For this review, use the dimensioned drawing (mm, ordinates from the lowest corner) and the shaded views. A direction names the side the tool comes from. Coordinates: 2 decimals unless noted, no trailing zeros. Loops run counter-clockwise (first coordinate to the right, second up) from the corner with the lowest first, then second, coordinate; pieces in that order, holes last. Notation, with made-up numbers: (63, 47.5) - (111, 47.5) arc R28 cw to (111, 82.5) - close; hole circle Ø1 at (88.25, -8.75). An arc over 180 degrees is marked (long way). Use a Markdown table: item, result. Add a question column.
1) The part is to be moulded in two halves that separate along X. For the marked faces 1, 2 and 3, say which applies: pulls with the +X half, pulls with the -X half, needs draft (parallel to the pull), parting line crosses it, or undercut.
2) Add section C-C, the plane z = 8. Give the boundary of the cut face in (x, y), and give its area (3 significant figures).
3) Add section B-B, the plane y = 30. Give the boundary of the cut face in (x, z).
4) Add section D-D, the plane z = 21. Give the boundary of the cut face in (x, y).
5) Clearance check with flat-ended pins moving along their axes: pin 1 (5 mm diameter, centred on y = 25, z = 8, fed in from -X); pin 2 (4 mm diameter, centred on x = 18, z = 28, fed in from +Y); pin 3 (1.6 mm diameter, centred on y = 32, z = 1, fed in from -X). State where each tip first meets the part, or that it passes through.
6) For the marked faces 4 and 5, list the 3-axis set-ups (+Z, -Z, +X, -X, +Y, -Y) from which the entire face can be reached by the end or side of a thin tool; tool diameter is ignored.
7) To check wall thickness, follow L1, parallel to Z at x = 24.5, y = 24; L2, parallel to X at y = 36.5, z = 6; L3, parallel to Z at x = 30.5, y = 57. State the ranges of each line that lie inside material, in increasing order. Write a range as [from, to].
8) Add section A-A, the plane x = 30. Give the boundary of the cut face in (y, z).
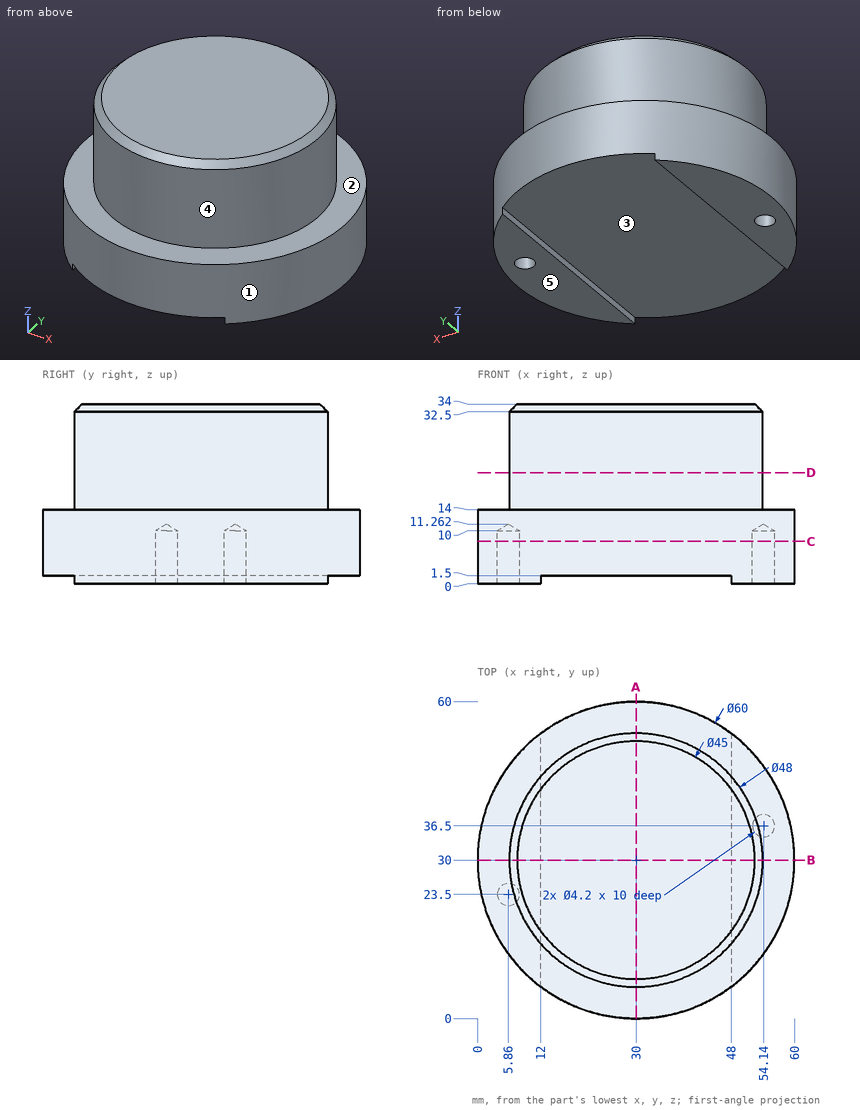
From the geometry:
| question | item | result |
|---|---|---|
| 1 | face 1 | parting line crosses it |
| 1 | face 2 | needs draft |
| 1 | face 3 | undercut |
| 2 | outline | circle Ø60 at (30, 30); hole circle Ø4.2 at (5.86, 23.5); hole circle Ø4.2 at (54.14, 36.5) |
| 2 | area | 2,800 mm^2 |
| 3 | outline | (0, 0) - (12, 0) - (12, 1.5) - (48, 1.5) - (48, 0) - (60, 0) - (60, 14) - (54, 14) - (54, 32.5) - (52.5, 34) - (7.5, 34) - (6, 32.5) - (6, 14) - (0, 14) - close |
| 4 | outline | circle Ø48 at (30, 30) |
| 5 | pin 1 | stops at x = 0.1 |
| 5 | pin 2 | stops at y = 51.82 |
| 5 | pin 3 | stops at x = 0.02 |
| 6 | face 4 | +Z |
| 6 | face 5 | -Z, +X, -X, +Y, -Y |
| 7 | L1 | z = [1.5, 34] |
| 7 | L2 | x = [0.71, 52.04], [56.24, 59.29] |
| 7 | L3 | z = [1.5, 14] |
| 8 | outline | (0, 1.5) - (60, 1.5) - (60, 14) - (54, 14) - (54, 32.5) - (52.5, 34) - (7.5, 34) - (6, 32.5) - (6, 14) - (0, 14) - close |
